Verification items for the finished model (mm, model axes). Coordinates: 2 decimals unless noted, no trailing zeros. Order: outer loops, then holes, each group sorted by start corner. A loop starts at its lowest first (then second) coordinate and runs counter-clockwise, first axis right, second up. Notation, with made-up numbers: M -8.75,20.25 L 10.25,20.25 A7 cw 10.25,32.25 Z; hole C -27.5,31 d8. An arc over 180 degrees is marked long. Return JSON: item names as keys, results as strings.
```python
from build123d import *

# Parameters (mm, degrees)
F0_R     = 11
F1_DEPTH = 50
F2_R     = 11
F3_T     = -2


with BuildPart() as f1:
    # F0 (on Top) → F1 (new body, symmetric)
    with BuildSketch(Plane.XY):
        Circle(F0_R)
    extrude(amount=F1_DEPTH, both=True)

    # F2
    f2_edges = [f1.edges().sort_by_distance(p)[0] for p in [
        (-11, 0, 50),
    ]]
    fillet(f2_edges, radius=F2_R)

    # F3
    f3_openings = [f1.faces().sort_by_distance(p)[0] for p in [
        (0, 0, -50),
    ]]
    offset(amount=F3_T, openings=f3_openings)


solid = f1.part
```
Q1. Draft check along X on faces 1 (the face through (-2.38, -10.74, -4.88)), 2 (the face through (2, -9, -50)), 3 (the face through (-1.172, 8.923, -4.877)). Enter one of: pulls with the +X half, pulls with the -X half, needs draft (parallel to the pull), parting line crosses it, or undercut.
Values:
{"face 1": "parting line crosses it", "face 2": "needs draft", "face 3": "undercut"}
Q2. Material ranges on line 1 along Y through (x, z) = (0, -7); line 2 along X through (y, z) = (-7.75, -38); line 3 along X through (y, z) = (5.25, 22.5), recorded low to high.
Values:
{"line 1": "-11 to -9, 9 to 11", "line 2": "-7.81 to -4.58, 4.58 to 7.81", "line 3": "-9.67 to -7.31, 7.31 to 9.67"}
Q3. Go/stop test with flat-tipped pins: pin 1 (1.5 mm diameter, centred on x = 6, z = 3, fed in from -Y); pin 2 (2 mm diameter, centred on y = -2.5, z = -0.5, fed in from +X); pin 3 (8 mm diameter, centred on y = 7, z = 23, fed in from -X). Record where each tip stops, or that it passes through.
Values:
{"pin 1": "y = -9.67", "pin 2": "x = 10.9", "pin 3": "x = -10.58"}
Q4. Cross-section at A-A, the plane x = 0. Record the boundary of the cut face in (y, z).
Values:
{"outline": "M -11,-50 L -9,-50 L -9,39 A9 cw 9,39 L 9,-50 L 11,-50 L 11,39 A11 ccw -11,39 Z"}
Q5. Cross-section at C-C, the plane z = 12. Record the boundary of the cut face in (x, y).
Values:
{"outline": "C 0,0 d22; hole C 0,0 d18"}
